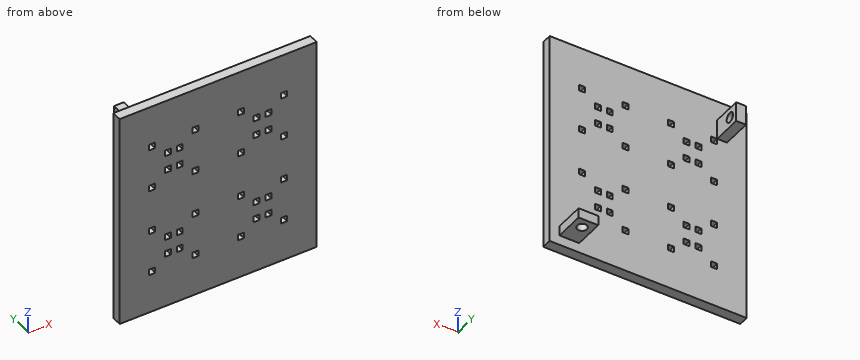
from build123d import *

# Parameters (mm, degrees)
SKETCH1_W           = 100
SKETCH1_H           = 110
SKETCH1_W_2         = 3
SKETCH1_H_2         = 3
BOSS_EXTRUDE1_DEPTH = 5
SKETCH2_W           = 10
SKETCH2_H           = 5
SKETCH2_W_2         = 5
SKETCH2_H_2         = 10
BOSS_EXTRUDE2_DEPTH = 15
SKETCH3_R           = 2.5
CUT_EXTRUDE1_DEPTH  = 15
SKETCH5_R           = 2.5
CUT_EXTRUDE2_DEPTH  = 15


with BuildPart() as part:
    # Sketch1 → Boss-Extrude1 (new body)
    with BuildSketch(Plane(origin=(0, 0, 0), x_dir=(1, 0, 0), z_dir=(0, 1, 0))):
        with Locations((-50, 55)):
            Rectangle(SKETCH1_W, SKETCH1_H)
        with Locations((-38.5, 43.5)):
            Rectangle(SKETCH1_W_2, SKETCH1_H_2, mode=Mode.SUBTRACT)
        with Locations((-16.5, 43.5)):
            Rectangle(SKETCH1_W_2, SKETCH1_H_2, mode=Mode.SUBTRACT)
        with Locations((-38.5, 21.5)):
            Rectangle(SKETCH1_W_2, SKETCH1_H_2, mode=Mode.SUBTRACT)
        with Locations((-16.5, 21.5)):
            Rectangle(SKETCH1_W_2, SKETCH1_H_2, mode=Mode.SUBTRACT)
        with Locations((-30.5, 37)):
            Rectangle(SKETCH1_W_2, SKETCH1_H_2, mode=Mode.SUBTRACT)
        with Locations((-30.5, 28)):
            Rectangle(SKETCH1_W_2, SKETCH1_H_2, mode=Mode.SUBTRACT)
        with Locations((-24.5, 37)):
            Rectangle(SKETCH1_W_2, SKETCH1_H_2, mode=Mode.SUBTRACT)
        with Locations((-24.5, 28)):
            Rectangle(SKETCH1_W_2, SKETCH1_H_2, mode=Mode.SUBTRACT)
        with Locations((-75.5, 28)):
            Rectangle(SKETCH1_W_2, SKETCH1_H_2, mode=Mode.SUBTRACT)
        with Locations((-75.5, 37)):
            Rectangle(SKETCH1_W_2, SKETCH1_H_2, mode=Mode.SUBTRACT)
        with Locations((-69.5, 28)):
            Rectangle(SKETCH1_W_2, SKETCH1_H_2, mode=Mode.SUBTRACT)
        with Locations((-69.5, 37)):
            Rectangle(SKETCH1_W_2, SKETCH1_H_2, mode=Mode.SUBTRACT)
        with Locations((-83.5, 21.5)):
            Rectangle(SKETCH1_W_2, SKETCH1_H_2, mode=Mode.SUBTRACT)
        with Locations((-61.5, 21.5)):
            Rectangle(SKETCH1_W_2, SKETCH1_H_2, mode=Mode.SUBTRACT)
        with Locations((-83.5, 43.5)):
            Rectangle(SKETCH1_W_2, SKETCH1_H_2, mode=Mode.SUBTRACT)
        with Locations((-61.5, 43.5)):
            Rectangle(SKETCH1_W_2, SKETCH1_H_2, mode=Mode.SUBTRACT)
        with Locations((-61.5, 66.5)):
            Rectangle(SKETCH1_W_2, SKETCH1_H_2, mode=Mode.SUBTRACT)
        with Locations((-83.5, 66.5)):
            Rectangle(SKETCH1_W_2, SKETCH1_H_2, mode=Mode.SUBTRACT)
        with Locations((-61.5, 88.5)):
            Rectangle(SKETCH1_W_2, SKETCH1_H_2, mode=Mode.SUBTRACT)
        with Locations((-83.5, 88.5)):
            Rectangle(SKETCH1_W_2, SKETCH1_H_2, mode=Mode.SUBTRACT)
        with Locations((-69.5, 73)):
            Rectangle(SKETCH1_W_2, SKETCH1_H_2, mode=Mode.SUBTRACT)
        with Locations((-69.5, 82)):
            Rectangle(SKETCH1_W_2, SKETCH1_H_2, mode=Mode.SUBTRACT)
        with Locations((-75.5, 73)):
            Rectangle(SKETCH1_W_2, SKETCH1_H_2, mode=Mode.SUBTRACT)
        with Locations((-75.5, 82)):
            Rectangle(SKETCH1_W_2, SKETCH1_H_2, mode=Mode.SUBTRACT)
        with Locations((-24.5, 82)):
            Rectangle(SKETCH1_W_2, SKETCH1_H_2, mode=Mode.SUBTRACT)
        with Locations((-24.5, 73)):
            Rectangle(SKETCH1_W_2, SKETCH1_H_2, mode=Mode.SUBTRACT)
        with Locations((-30.5, 82)):
            Rectangle(SKETCH1_W_2, SKETCH1_H_2, mode=Mode.SUBTRACT)
        with Locations((-30.5, 73)):
            Rectangle(SKETCH1_W_2, SKETCH1_H_2, mode=Mode.SUBTRACT)
        with Locations((-16.5, 88.5)):
            Rectangle(SKETCH1_W_2, SKETCH1_H_2, mode=Mode.SUBTRACT)
        with Locations((-38.5, 88.5)):
            Rectangle(SKETCH1_W_2, SKETCH1_H_2, mode=Mode.SUBTRACT)
        with Locations((-16.5, 66.5)):
            Rectangle(SKETCH1_W_2, SKETCH1_H_2, mode=Mode.SUBTRACT)
        with Locations((-38.5, 66.5)):
            Rectangle(SKETCH1_W_2, SKETCH1_H_2, mode=Mode.SUBTRACT)
    extrude(amount=BOSS_EXTRUDE1_DEPTH)

    # Sketch2 → Boss-Extrude2 (add)
    with BuildSketch(Plane(origin=(0, 5, 0), x_dir=(1, 0, 0), z_dir=(0, 1, 0))):
        with Locations((-10, 102.5)):
            Rectangle(SKETCH2_W, SKETCH2_H)
        with Locations((-87.5, 15)):
            Rectangle(SKETCH2_W_2, SKETCH2_H_2)
    extrude(amount=BOSS_EXTRUDE2_DEPTH)

    # Sketch3 → Cut-Extrude1 (cut)
    with BuildSketch(Plane(origin=(0, 0, -105), x_dir=(-1, 0, 0), z_dir=(0, 0, -1))):
        with Locations((10, 15)):
            Circle(SKETCH3_R)
    extrude(amount=-CUT_EXTRUDE1_DEPTH, mode=Mode.SUBTRACT)

    # Sketch5 → Cut-Extrude2 (cut)
    with BuildSketch(Plane.ZY.offset(90)):
        with Locations((-15, 15)):
            Circle(SKETCH5_R)
    extrude(amount=-CUT_EXTRUDE2_DEPTH, mode=Mode.SUBTRACT)


solid = part.part
Input: part model. Units: mm. Frame: model coordinates. Give positions to 0.01 mm unless a question says otherwise; leave off trailing zeros. Order: outer loops, then holes, each group sorted by start corner. A loop starts at its lowest first (then second) coordinate and runs counter-clockwise, first axis right, second up. Notation, with made-up numbers: (-16.5, -30) - (16.5, -30) arc R19 cw to (16.5, -20) - close; hole circle Ø10 at (-23, -6). An arc over 180 degrees is marked (long way). Answer as a JSON object with one key per item and string values. Group by question number.
Q1. Line query: probe 1 along X at (y, z) = (2.75, -73); probe 2 along Z at (x, y) = (-23.5, 3.5); probe 3 along Y at (x, z) = (-10, -102). Output: solid intervals per line, ascending.
Q2. Cut plane D-D, the plane y = 9.5. Output: boundary loops of the cut face in (x, z), then the cut area to 3 significant figures.
Q3. Cut plane B-B, the plane y = 15. Output: boundary loops of the cut face in (x, z), then the cut area to 3 significant figures.
Q4. Cut plane A-A, the plane x = -10. Output: boundary loops of the cut face in (y, z), then the cut area to 3 significant figures.
Q5. First-contact query: pin 1 Ø3.5 at (x, y) = (-75.5, 2) entering from +Z; pin 2 Ø6 at (x, z) = (-74.5, -82.5) entering from +Y; pin 3 Ø5 at (x, y) = (-16.5, 10) entering from +Z; pin 4 Ø2.5 at (x, y) = (-88, 14.5) entering from -Z. Flat tips, straight axial feed; report the tip coordinate or a pass-through.
Q6. Cut plane C-C, the plane z = -15. Output: boundary loops of the cut face in (x, y), then the cut area to 3 significant figures.
Results:
{
 "1": {"probe 1": "-100 to -77, -74 to -71, -68 to -32, -29 to -26, -23 to 0", "probe 2": "-110 to -83.5, -80.5 to -74.5, -71.5 to -38.5, -35.5 to -29.5, -26.5 to 0", "probe 3": "0 to 12.5, 17.5 to 20"},
 "2": {"outline": "(-90, -20) - (-85, -20) - (-85, -10) - (-90, -10) - close; (-15, -105) - (-5, -105) - (-5, -100) - (-15, -100) - close", "area": "100 mm^2"},
 "3": {"outline": "(-90, -20) - (-85, -20) - (-85, -17.5) - (-90, -17.5) - close; (-90, -12.5) - (-85, -12.5) - (-85, -10) - (-90, -10) - close; (-15, -105) - (-12.5, -105) - (-12.5, -100) - (-15, -100) - close; (-7.5, -105) - (-5, -105) - (-5, -100) - (-7.5, -100) - close", "area": "50.0 mm^2"},
 "4": {"outline": "(0, -110) - (5, -110) - (5, -105) - (12.5, -105) - (12.5, -100) - (5, -100) - (5, 0) - (0, 0) - close; (17.5, -105) - (20, -105) - (20, -100) - (17.5, -100) - close", "area": "600 mm^2"},
 "5": {"pin 1": "z = 0", "pin 2": "y = 5", "pin 3": "z = -100", "pin 4": "z = -20"},
 "6": {"outline": "(-100, 0) - (0, 0) - (0, 5) - (-85, 5) - (-85, 12.5) - (-90, 12.5) - (-90, 5) - (-100, 5) - close; (-90, 17.5) - (-85, 17.5) - (-85, 20) - (-90, 20) - close", "area": "550 mm^2"}
}
